Part model, mm, in its own coordinate system. A direction names the side the tool comes from. Coordinates: 2 decimals unless noted, no trailing zeros. Loops run counter-clockwise (first coordinate to the right, second up) from the corner with the lowest first, then second, coordinate; pieces in that order, holes last. Notation, with made-up numbers: M 18.25,81 L 77.25,81 A18 cw 77.25,97 Z; hole C 9,49 d4. An arc over 180 degrees is marked long. Answer as a JSON object with one key per item and string values. Group by question number.
1. Drill centre lines: L1, parallel to X at y = -91, z = 11 (3 decimals); L2, parallel to X at y = -106, z = 19.5 (3 decimals); L3, parallel to Z at x = -1.75, y = -45.5. Where is each one in solid material? Low to high.
2. Mould opens along X. For faces 5 (the face through (-17.745, -64, 20)), 6 (the face through (-14.495, -64, 20)), 7 (the face through (-14.495, -64, 28)), 8 (the face through (-7, -64, 25)) say: released by +X, released by -X, zero draft, split by the parting line, or undercut.
3. Drop flat-ended pins along their axis: pin 1 Ø1 at (x, y) = (-9.5, -65) entering from +Z; pin 2 Ø1.5 at (y, z) = (-82, 27.5) entering from -X (3 decimals); pin 3 Ø1.1 at (x, y) = (-16.5, -62) entering from -Z. Give the stop position or say it passes through.
4. 3-axis set-ups, long thin cutter, end or side, ignore diameter. For faces 1 (the face through (0, -64, 12)), 2 (the face through (-8, 0, 17)), 3 (the face through (-21, -64, 23)), 4 (the face through (-6.995, -64, 11)): which of +Z, -Z, +X, -X, +Y, -Y reach the whole face in a straight line?
5. Saw through at C-C on x = -21. Write the cut outline in (y, z).
6. Saw through at A-A on z = 12. Write the cut outline in (x, y) (3 decimals).
from build123d import *

# Parameters (mm, degrees)
F1_DEPTH = 130


with BuildPart() as f1:
    # F0 (on Front) → F1 (new body)
    with BuildSketch(Plane.XZ):
        with BuildLine():
            Line((-2, 0), (0, 0))
            Line((0, 0), (0, 24.5))
            ThreePointArc((0, 24.5), (-0.146447, 24.853553), (-0.5, 25))
            Line((-0.5, 25), (-13.995, 25))
            ThreePointArc((-13.995, 25), (-14.348553, 25.146447), (-14.495, 25.5))
            Line((-14.495, 25.5), (-14.495, 30.5))
            ThreePointArc((-14.495, 30.5), (-14.641447, 30.853553), (-14.995, 31))
            Line((-14.995, 31), (-17.245, 31))
            ThreePointArc((-17.245, 31), (-17.598553, 30.853553), (-17.745, 30.5))
            Line((-17.745, 30.5), (-17.745, 25.5))
            ThreePointArc((-17.745, 25.5), (-17.891447, 25.146447), (-18.245, 25))
            Line((-18.245, 25), (-24.25953, 25))
            ThreePointArc((-24.25953, 25), (-24.754721, 24.991876), (-25, 24.561623))
            Line((-25, 24.561623), (-25, 23.5))
            ThreePointArc((-25, 23.5), (-24.853553, 23.146447), (-24.5, 23))
            Line((-24.5, 23), (-18.245, 23))
            ThreePointArc((-18.245, 23), (-17.891447, 22.853553), (-17.745, 22.5))
            Line((-17.745, 22.5), (-17.745, 17.5))
            ThreePointArc((-17.745, 17.5), (-17.598553, 17.146447), (-17.245, 17))
            Line((-17.245, 17), (-14.995, 17))
            ThreePointArc((-14.995, 17), (-14.641447, 17.146447), (-14.495, 17.5))
            Line((-14.495, 17.5), (-14.495, 22.5))
            ThreePointArc((-14.495, 22.5), (-14.348553, 22.853553), (-13.995, 23))
            Line((-13.995, 23), (-9.495, 23))
            ThreePointArc((-9.495, 23), (-9.141447, 22.853553), (-8.995, 22.5))
            Line((-8.995, 22.5), (-8.995, 0))
            Line((-8.995, 0), (-6.995, 0))
            Line((-6.995, 0), (-6.995, 22.5))
            ThreePointArc((-6.995, 22.5), (-6.848553, 22.853553), (-6.495, 23))
            Line((-6.495, 23), (-2.5, 23))
            ThreePointArc((-2.5, 23), (-2.146447, 22.853553), (-2, 22.5))
            Line((-2, 22.5), (-2, 0))
        make_face()
    extrude(amount=F1_DEPTH)


solid = f1.part
Outcome:
{
 "1": {"L1": "x = -8.995 to -6.995, -2 to 0", "L2": "x = -17.745 to -14.495, -8.995 to -6.995, -2 to 0", "L3": "z = 0 to 25"},
 "2": {"face 5": "released by -X", "face 6": "undercut", "face 7": "released by +X", "face 8": "zero draft"},
 "3": {"pin 1": "stops at z = 25", "pin 2": "stops at x = -17.745", "pin 3": "stops at z = 17"},
 "4": {"face 1": "+Z, -Z, +X, +Y, -Y", "face 2": "+Z, -Z, +X, -X, +Y", "face 3": "-Z, -X, +Y, -Y", "face 4": "-Z, +Y, -Y"},
 "5": {"outline": "M -130,23 L 0,23 L 0,25 L -130,25 Z"},
 "6": {"outline": "M -8.995,-130 L -6.995,-130 L -6.995,0 L -8.995,0 Z; M -2,-130 L 0,-130 L 0,0 L -2,0 Z"}
}
